Part print with two shaded views. Sizes in mm from the minimum x, y, z corner. A direction names the side the tool comes from. Coordinates: 2 decimals unless noted, no trailing zeros. Loops run counter-clockwise (first coordinate to the right, second up) from the corner with the lowest first, then second, coordinate; pieces in that order, holes last. Notation, with made-up numbers: (-12, -19) -> (-1, -19) arc R18 ccw to (-1, 1) -> close; hole circle Ø10 at (18, 46). An arc over 180 degrees is marked (long way). Answer as a JSON object with one key per item and string values. Group by question number.
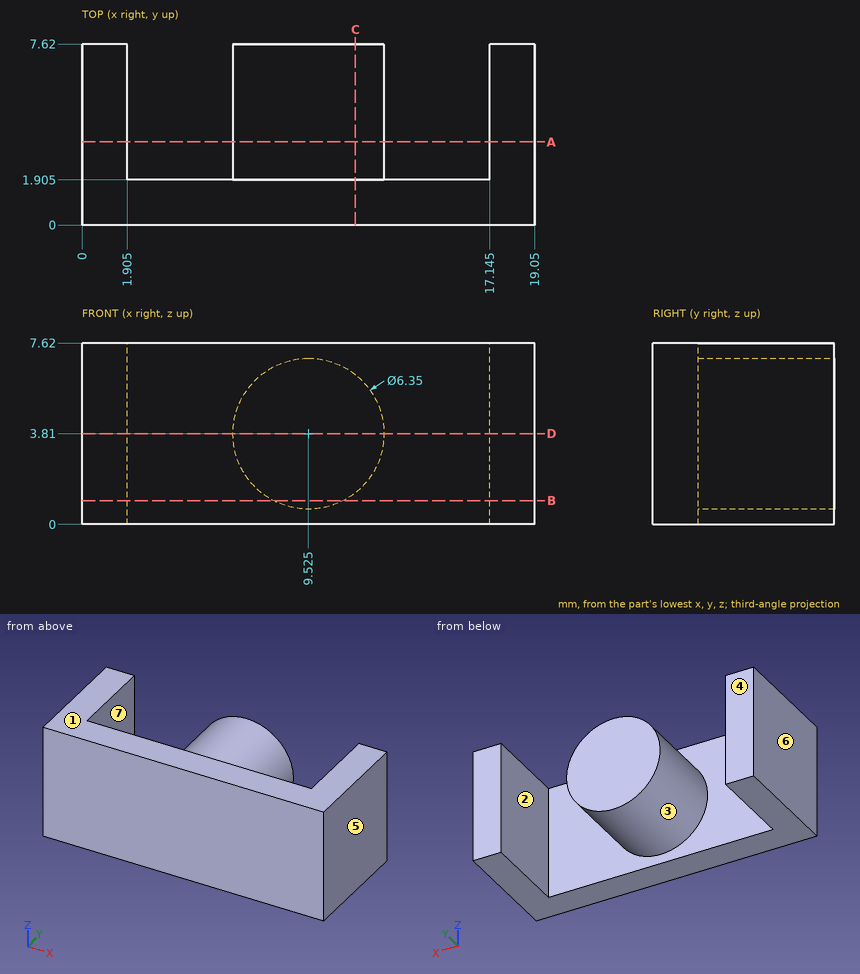
Item 1: Band-saw the part on A-A, the plane y = 3.5. List the corners of the cut face in (x, z) (3 decimals), and give its area (3 significant figures).
Item 2: Band-saw the part on D-D, the plane z = 3.81. List the corners of the cut face in (x, y) (3 decimals).
Item 3: Drill centre lines: L1, parallel to X at y = 6, z = 4.75 (3 decimals); L2, parallel to X at y = 5.75, z = 0.5 (3 decimals); L3, parallel to X at y = 2.75, z = 1.5 (3 decimals). Where is each one in solid material? Low to high.
Item 4: Band-saw the part on C-C, the plane x = 11.5. List the corners of the cut face in (y, z) (3 decimals).
Item 5: Flat gauge pins, fed straight in: P1, Ø2, axis at x = 5, y = 5, coming from the -Z side; P2, Ø4, axis at x = 6.5, y = 5.5, coming from the -Z side (3 decimals). Where does each tip first touch, or does it go through?
Item 6: Pull direction X, two halves, no side cores. Call the marked faces 4, 5, 6 and 7: +X half, -X half, draft (parallel to the pull), parting line (faces both ways), or undercut.
Item 7: Band-saw the part on B-B, the plane z = 1. List the corners of the cut face in (x, y) (3 decimals), and give its area (3 significant figures).
Item 8: 3-axis set-ups, long thin cutter, end or side, ignore diameter. For the marked faces 1, 2 and 3: which of +Z, -Z, +X, -X, +Y, -Y reach the whole face in a straight line?
Reply:
{
 "1": {"outline": "(0, 0) -> (1.905, 0) -> (1.905, 7.62) -> (0, 7.62) -> close; circle Ø6.35 at (9.525, 3.81); (17.145, 0) -> (19.05, 0) -> (19.05, 7.62) -> (17.145, 7.62) -> close", "area": "60.7 mm²"},
 "2": {"outline": "(0, 0) -> (19.05, 0) -> (19.05, 7.62) -> (17.145, 7.62) -> (17.145, 1.905) -> (12.7, 1.905) -> (12.7, 7.62) -> (6.35, 7.62) -> (6.35, 1.905) -> (1.905, 1.905) -> (1.905, 7.62) -> (0, 7.62) -> close"},
 "3": {"L1": "0 to 1.905, 6.492 to 12.558, 17.145 to 19.05", "L2": "0 to 1.905, 17.145 to 19.05", "L3": "0 to 1.905, 7.347 to 11.703, 17.145 to 19.05"},
 "4": {"outline": "(0, 0) -> (1.905, 0) -> (1.905, 1.324) -> (7.62, 1.324) -> (7.62, 6.296) -> (1.905, 6.296) -> (1.905, 7.62) -> (0, 7.62) -> close"},
 "5": {"P1": "through", "P2": "z = 0.805"},
 "6": {"face 4": "draft", "face 5": "+X half", "face 6": "-X half", "face 7": "undercut"},
 "7": {"outline": "(0, 0) -> (19.05, 0) -> (19.05, 7.62) -> (17.145, 7.62) -> (17.145, 1.905) -> (11.003, 1.905) -> (11.003, 7.62) -> (8.047, 7.62) -> (8.047, 1.905) -> (1.905, 1.905) -> (1.905, 7.62) -> (0, 7.62) -> close", "area": "75.0 mm²"},
 "8": {"face 1": "+Z, +X, -X, +Y, -Y", "face 2": "+Z, -Z, +Y", "face 3": "+Y"}
}
